CAD build for the part. Positions are in the model's coordinates, mm. A direction names the side the tool comes from. Round coordinates to 2 decimals unless told otherwise and drop trailing zeros. Write each loop counter-clockwise with the first axis right and the second up, starting at its lowest first coordinate (ties: lowest second). Pieces come first, ordered by that corner, then holes. Notation, with made-up numbers: (-32, 54.25) - (10, 54.25) arc R12 cw to (10, 73.25) - close; hole circle Ø5 at (-32.5, -32). An arc over 180 degrees is marked (long way). Answer in a Markdown table with one row per item.
```python
from build123d import *

# Parameters (mm, degrees)
F0_W      = 228.6
F0_H      = 76.2
F1_DEPTH  = 12.7
F2_W      = 173.19999904
F2_H      = 22.19999878
F3_DEPTH  = 7.62
F4_R      = 10.795
F5_DEPTH  = 6.35
F7_DEPTH  = 6.35
F8_R      = 2.0066
F9_DEPTH  = 9.652
F10_R     = 2.0066
F11_DEPTH = 9.652
F12_R     = 2.921
F13_DEPTH = 2.5019
F14_R     = 2.921
F15_DEPTH = 2.5019
F16_R     = 5.08
F18_DEPTH = 2.50000008
F19_R     = 1.2446
F21_DEPTH = 1.27


with BuildPart() as f1:
    # F0 (on Top) → F1 (new body)
    with BuildSketch(Plane.XY):
        Rectangle(F0_W, F0_H)
    extrude(amount=F1_DEPTH)

    # F2 (on face) → F3 (cut)
    with BuildSketch(Plane.XY.offset(12.7)):
        Rectangle(F2_W, F2_H)
    extrude(amount=-F3_DEPTH, mode=Mode.SUBTRACT)

    # F4 (on face) → F5 (cut)
    with BuildSketch(Plane.XY.offset(12.7)):
        with Locations((-86.59999952, 0)):
            Circle(F4_R)
        with Locations((86.59999952, 0)):
            Circle(F4_R)
    extrude(amount=-F5_DEPTH, mode=Mode.SUBTRACT)

    # F6 (on face) → F7 (cut)
    with BuildSketch(Plane.XY.offset(12.7)):
        with BuildLine():
            Line((-75.80499952, -11.09999939), (-86.59999952, -11.09999939))
            ThreePointArc((-86.59999952, -11.09999939), (-75.80499952, -21.89499939), (-65.00999952, -11.09999939))
            Line((-65.00999952, -11.09999939), (-75.80499952, -11.09999939))
        make_face()
        with BuildLine():
            ThreePointArc((86.59999952, 11.09999939), (75.80499952, 21.89499939), (65.00999952, 11.09999939))
            Line((65.00999952, 11.09999939), (75.80499952, 11.09999939))
            Line((75.80499952, 11.09999939), (86.59999952, 11.09999939))
        make_face()
        with BuildLine():
            Line((75.80499952, -11.09999939), (65.00999952, -11.09999939))
            ThreePointArc((65.00999952, -11.09999939), (75.80499952, -21.89499939), (86.59999952, -11.09999939))
            Line((86.59999952, -11.09999939), (75.80499952, -11.09999939))
        make_face()
        with BuildLine():
            ThreePointArc((-65.00999952, 11.09999939), (-75.80499952, 21.89499939), (-86.59999952, 11.09999939))
            Line((-86.59999952, 11.09999939), (-75.80499952, 11.09999939))
            Line((-75.80499952, 11.09999939), (-65.00999952, 11.09999939))
        make_face()
    extrude(amount=-F7_DEPTH, mode=Mode.SUBTRACT)

    # F8 (on face) → F9 (cut)
    with BuildSketch(Plane(origin=(-114.3, 0, 0), x_dir=(0, -1, 0), z_dir=(-1, 0, 0))):
        with Locations((0, 6.35)):
            Circle(F8_R)
    extrude(amount=-F9_DEPTH, mode=Mode.SUBTRACT)

    # F10 (on face) → F11 (cut)
    with BuildSketch(Plane.YZ.offset(114.3)):
        with Locations((0, 6.35)):
            Circle(F10_R)
    extrude(amount=-F11_DEPTH, mode=Mode.SUBTRACT)

    # F12 (on face) → F13 (cut)
    with BuildSketch(Plane(origin=(-114.3, 0, 0), x_dir=(0, -1, 0), z_dir=(-1, 0, 0))):
        with Locations((-25.4, 6.35)):
            Circle(F12_R)
        with Locations((25.4, 6.35)):
            Circle(F12_R)
    extrude(amount=-F13_DEPTH, mode=Mode.SUBTRACT)

    # F14 (on face) → F15 (cut)
    with BuildSketch(Plane.YZ.offset(114.3)):
        with Locations((-25.4, 6.35)):
            Circle(F14_R)
        with Locations((25.4, 6.35)):
            Circle(F14_R)
    extrude(amount=-F15_DEPTH, mode=Mode.SUBTRACT)

    # F16 (call 1 of 6: OpenCascade refuses the feature's edges together)
    f16_edges = [f1.edges().sort_by_distance(p)[0] for p in [
        (-97.395, 0, 6.35),
    ]]
    fillet(f16_edges, radius=F16_R)

    # F16#2 (call 2 of 6)
    f16_2_edges = [f1.edges().sort_by_distance(p)[0] for p in [
        (-75.805, 21.894999, 6.35),
    ]]
    fillet(f16_2_edges, radius=F16_R)

    # F16#3 (call 3 of 6)
    f16_3_edges = [f1.edges().sort_by_distance(p)[0] for p in [
        (-75.805, -21.894999, 6.35),
    ]]
    fillet(f16_3_edges, radius=F16_R)

    # F16#4 (call 4 of 6)
    f16_4_edges = [f1.edges().sort_by_distance(p)[0] for p in [
        (75.805, 21.894999, 6.35),
    ]]
    fillet(f16_4_edges, radius=F16_R)

    # F16#5 (call 5 of 6)
    f16_5_edges = [f1.edges().sort_by_distance(p)[0] for p in [
        (97.395, 0, 6.35),
    ]]
    fillet(f16_5_edges, radius=F16_R)

    # F16#6 (call 6 of 6)
    f16_6_edges = [f1.edges().sort_by_distance(p)[0] for p in [
        (75.805, -21.894999, 6.35),
    ]]
    fillet(f16_6_edges, radius=F16_R)

    # F17 (on face) → F18 (join)
    with BuildSketch(Plane.XY.offset(5.08)):
        with BuildLine():
            Line((-74.5000034, 8.25000001), (-74.5000034, 9.50000005))
            ThreePointArc((-74.5000034, 9.50000005), (-75.3838869048, 7.3661165052), (-73.25000336, 8.25000001))
            Line((-73.25000336, 8.25000001), (-74.5000034, 8.25000001))
        make_face()
        with BuildLine():
            ThreePointArc((-73.25000336, 8.25000001), (-73.6161198952, 9.1338835148), (-74.5000034, 9.50000005))
            Line((-74.5000034, 9.50000005), (-74.5000034, 8.25000001))
            Line((-74.5000034, 8.25000001), (-73.25000336, 8.25000001))
        make_face()
    extrude(amount=F18_DEPTH)

    # F19
    f19_edges = [f1.edges().sort_by_distance(p)[0] for p in [
        (-75.750003, 8.25, 7.58),
    ]]
    fillet(f19_edges, radius=F19_R)

    # F20 (on face) → F21 (cut)
    with BuildSketch(Plane.XY.offset(12.7)):
        with BuildLine():
            ThreePointArc((-86.59999952, 11.09999939), (-86.5987382997, 11.2650089547), (-86.5949549334, 11.429979962))
            ThreePointArc((-86.5949549334, 11.429979962), (-87.0538068899, 11.2391664903), (-87.2347248066, 10.7763235294))
            ThreePointArc((-87.2347248066, 10.7763235294), (-86.91749952, 10.7903298722), (-86.59999952, 10.795))
            Line((-86.59999952, 10.795), (-86.59999952, 11.09999939))
        make_face()
        with BuildLine():
            ThreePointArc((-86.59999952, -10.795), (-86.91749952, -10.7903298722), (-87.2347248066, -10.7763235294))
            ThreePointArc((-87.2347248066, -10.7763235294), (-87.0538068899, -11.2391664903), (-86.5949549334, -11.429979962))
            ThreePointArc((-86.5949549334, -11.429979962), (-86.5987382997, -11.2650089547), (-86.59999952, -11.09999939))
            Line((-86.59999952, -11.09999939), (-86.59999952, -10.795))
        make_face()
        with BuildLine():
            ThreePointArc((87.23499952, 10.795), (87.047225239, 11.2457928086), (86.5949549334, 11.429979962))
            ThreePointArc((86.5949549334, 11.429979962), (86.5987382997, 11.2650089547), (86.59999952, 11.09999939))
            Line((86.59999952, 11.09999939), (86.59999952, 10.795))
            ThreePointArc((86.59999952, 10.795), (86.91749952, 10.7903298722), (87.2347248066, 10.7763235294))
            ThreePointArc((87.2347248066, 10.7763235294), (87.2349308379, 10.7856607546), (87.23499952, 10.795))
        make_face()
        with BuildLine():
            ThreePointArc((87.23499952, -10.795), (87.2349308379, -10.7856607546), (87.2347248066, -10.7763235294))
            ThreePointArc((87.2347248066, -10.7763235294), (86.91749952, -10.7903298722), (86.59999952, -10.795))
            Line((86.59999952, -10.795), (86.59999952, -11.09999939))
            ThreePointArc((86.59999952, -11.09999939), (86.5987382997, -11.2650089547), (86.5949549334, -11.429979962))
            ThreePointArc((86.5949549334, -11.429979962), (87.047225239, -11.2457928086), (87.23499952, -10.795))
        make_face()
    extrude(amount=-F21_DEPTH, mode=Mode.SUBTRACT)


solid = f1.part
```
Q1. Saw through at A-A on x = -10. List the corners of the cut face in (y, z), then the cut area to 3 significant figures.
Computed:
| item | result |
|---|---|
| outline | (-38.1, 0) - (38.1, 0) - (38.1, 12.7) - (11.1, 12.7) - (11.1, 5.08) - (-11.1, 5.08) - (-11.1, 12.7) - (-38.1, 12.7) - close |
| area | 799 mm2 |
Q2. Pull direction X, two halves, no side cores. Call faces 4 (the cylindrical face through (-113.067, -23.247, 8.324)), 5 (the flat face through (-114.3, -1, 3)), 6 (the flat face through (-89, 0, 6.35)): released by +X, released by -X, zero draft, split by the parting line, or undercut.
Computed:
| item | result |
|---|---|
| face 4 | zero draft |
| face 5 | released by -X |
| face 6 | undercut |
Q3. 3-axis set-ups, long thin cutter, end or side, ignore diameter. For faces 1 (the cylindrical face through (-75.405, 21.888, 12.074)), 2 (the cylindrical face through (-109.54, -1.08, 8.04)), 3 (the cylindrical face through (113.067, -25.78, 9.246)): which of +Z, -Z, +X, -X, +Y, -Y reach the whole face in a straight line?
Computed:
| item | result |
|---|---|
| face 1 | +Z |
| face 2 | -X |
| face 3 | +X |
Q4. Drill centre lines: line 1 (X direction, y = -11.5, z = 12); line 2 (Y direction, x = -87, z = 11); line 3 (Y direction, x = 65.5, z = 8.5). Where is each one in solid material? Low to high.
Computed:
| item | result |
|---|---|
| line 1 | x = -114.3 to -86.59, -65.02 to 65.02, 86.59 to 114.3 |
| line 2 | y = -38.1 to -10.77, 10.77 to 38.1 |
| line 3 | y = -38.1 to -11.1, 11.1 to 38.1 |
Q5. Saw through at B-B on y = 0. List the corners of the cut face in (x, z) (3 decimals).
Computed:
| item | result |
|---|---|
| outline | (-114.3, 0) - (114.3, 0) - (114.3, 4.343) - (104.648, 4.343) - (104.648, 8.357) - (114.3, 8.357) - (114.3, 12.7) - (97.395, 12.7) - (97.395, 11.43) arc R5.08 cw to (92.315, 6.35) - (86.6, 6.35) - (86.6, 5.08) - (-86.6, 5.08) - (-86.6, 6.35) - (-92.315, 6.35) arc R5.08 cw to (-97.395, 11.43) - (-97.395, 12.7) - (-114.3, 12.7) - (-114.3, 8.357) - (-104.648, 8.357) - (-104.648, 4.343) - (-114.3, 4.343) - close |
Q6. Flat gauge pins, fed straight in: pin 1 (3.5 mm diameter, centred on y = -25.4, z = 6.35, fed in from -X); pin 2 (3 mm diameter, centred on x = 77.5, y = -14.5, fed in from +Z); pin 3 (4.5 mm diameter, centred on x = -77.5, y = 15, fed in from +Z). Where does each tip first touch, or does it go through?
Computed:
| item | result |
|---|---|
| pin 1 | stops at x = -111.8 |
| pin 2 | stops at z = 6.35 |
| pin 3 | stops at z = 6.41 |
